from build123d import *

# Parameters (mm, degrees)
SKETCH1_R           = 4.6
BOSS_EXTRUDE1_DEPTH = 5


with BuildPart() as part:
    # Sketch1 → Boss-Extrude1 (new body)
    with BuildSketch(Plane(origin=(0, 0, 0), x_dir=(1, 0, 0), z_dir=(0, 1, 0))):
        Circle(SKETCH1_R)
        Polygon((-0.994976924, 2.402086785), (-2.402086785, 0.994976924), (-2.402086785, -0.994976924), (-0.994976924, -2.402086785), (0.994976924, -2.402086785), (2.402086785, -0.994976924), (2.402086785, 0.994976924), (0.994976924, 2.402086785), align=None, mode=Mode.SUBTRACT)
    extrude(amount=BOSS_EXTRUDE1_DEPTH)


solid = part.part
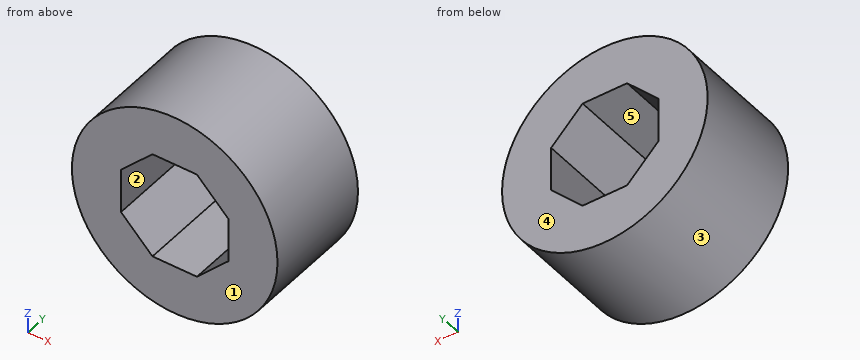
Input: part model. Units: mm. Frame: model coordinates. Face numbers are marked on the shaded views. A direction names the side the tool comes from. Coordinates: 2 decimals unless noted, no trailing zeros. Write each loop counter-clockwise with the first axis right and the second up, starting at its lowest first coordinate (ties: lowest second). Pieces come first, ordered by that corner, then holes. Notation, with made-up numbers: M 11,11 L 48,11 A24 ccw 48,42 Z; hole C -25,-36.5 d4. An arc over 180 degrees is marked long. Answer as a JSON object with one key per item and string values. Group by question number.
(1) Section D-D on x = -3.25. Output: boundary loops of the cut face in (y, z).
(2) Mould query, pull axis Z, two halves, no side actions, for the marked faces 1, 2 and 3. Classes: pulls with the +Z half, pulls with the -Z half, needs draft (parallel to the pull), parting line crosses it, or undercut.
(3) Section B-B on z = 0. Output: boundary loops of the cut face in (x, y).
(4) Section C-C on y = 1.05. Output: boundary loops of the cut face in (x, z), plus the area to 3 significant figures.
(5) Ray query, line 1 along X through (y, z) = (0.8, 0); line 2 along X through (y, z) = (2.1, -2). Return the intervals inside material, ascending. Write a range as [from, to].
(6) Section A-A on x = 0. Output: boundary loops of the cut face in (y, z), plus the area to 3 significant figures.
(7) Contact query for flat-ended pins moving along their axis: P1, Ø5, axis at x = -2, z = 1, coming from the -Y side; P2, Ø3, axis at y = 2.5, z = -3.5, coming from the -X side; P3, Ø2, axis at x = 2.5, y = 4, coming from the -Z side; P4, Ø0.6, axis at y = 1.5, z = 0.5, coming from the -X side. Output: stop coordinate, or through.
(8) Set-up query: the marked faces 4 and 5. Return all of +Z, -Z, +X, -X, +Y, -Y with unobstructed straight access to the full face (end or side cutting, diameter ignored); none if empty.
Result set:
{
 "1": {"outline": "M 0,-3.26 L 5,-3.26 L 5,3.26 L 0,3.26 Z"},
 "2": {"face 1": "needs draft", "face 2": "undercut", "face 3": "parting line crosses it"},
 "3": {"outline": "M -4.6,0 L -2.4,0 L -2.4,5 L -4.6,5 Z; M 2.4,0 L 4.6,0 L 4.6,5 L 2.4,5 Z"},
 "4": {"outline": "C 0,0 d9.2; hole M -2.4,-0.99 L -0.99,-2.4 L 0.99,-2.4 L 2.4,-0.99 L 2.4,0.99 L 0.99,2.4 L -0.99,2.4 L -2.4,0.99 Z", "area": "47.4 mm2"},
 "5": {"line 1": "x = [-4.6, -2.4], [2.4, 4.6]", "line 2": "x = [-4.14, -1.4], [1.4, 4.14]"},
 "6": {"outline": "M 0,-4.6 L 5,-4.6 L 5,-2.4 L 0,-2.4 Z; M 0,2.4 L 5,2.4 L 5,4.6 L 0,4.6 Z", "area": "22.0 mm2"},
 "7": {"P1": "stops at y = 0", "P2": "stops at x = -4.14", "P3": "stops at z = -4.35", "P4": "stops at x = -4.6"},
 "8": {"face 4": "+Z, -Z, +X, -X, +Y", "face 5": "+Y, -Y"}
}
